Part model, mm, in its own coordinate system. A direction names the side the tool comes from. Coordinates: 2 decimals unless noted, no trailing zeros. Write each loop counter-clockwise with the first axis right and the second up, starting at its lowest first coordinate (ties: lowest second). Pieces come first, ordered by that corner, then holes. Notation, with made-up numbers: (85, -0.75) - (89, -0.75) arc R19 cw to (89, 33.25) - close; hole circle Ø7 at (-27, -29.5). An arc over 180 degrees is marked (long way). Use a Markdown table: item, result.
```python
from build123d import *

# Parameters (mm, degrees)
F1_DEPTH      = 25
F1_DEPTH_BACK = 25
F2_SIZE2      = 5
F2_SIZE       = 1
F3_SIZE2      = 1
F3_SIZE       = 5
F3_2_SIZE2    = 1
F3_2_SIZE     = 5
F3_3_SIZE2    = 1
F3_3_SIZE     = 5
F3_4_SIZE2    = 1
F3_4_SIZE     = 5


with BuildPart() as f1:
    # F0 (on Front) → F1 (new body, two sides)
    with BuildSketch(Plane.XZ) as f1_sk:
        with BuildLine():
            Line((-1.5, -2), (-1.5, -6.0415747119))
            ThreePointArc((-1.5, -6.0415747119), (0, -6.225), (1.5, -6.0415747119))
            Line((1.5, -6.0415747119), (1.5, -2))
            ThreePointArc((1.5, -2), (1.767766953, -1.767766953), (2, -1.5))
            Line((2, -1.5), (6.0415747119, -1.5))
            ThreePointArc((6.0415747119, -1.5), (6.225, 0), (6.0415747119, 1.5))
            Line((6.0415747119, 1.5), (2, 1.5))
            ThreePointArc((2, 1.5), (1.767766953, 1.767766953), (1.5, 2))
            Line((1.5, 2), (1.5, 6.0415747119))
            ThreePointArc((1.5, 6.0415747119), (0, 6.225), (-1.5, 6.0415747119))
            Line((-1.5, 6.0415747119), (-1.5, 2))
            ThreePointArc((-1.5, 2), (-1.767766953, 1.767766953), (-2, 1.5))
            Line((-2, 1.5), (-6.0415747119, 1.5))
            ThreePointArc((-6.0415747119, 1.5), (-6.225, 0), (-6.0415747119, -1.5))
            Line((-6.0415747119, -1.5), (-2, -1.5))
            ThreePointArc((-2, -1.5), (-1.767766953, -1.767766953), (-1.5, -2))
        make_face()
    extrude(amount=F1_DEPTH)
    extrude(f1_sk.sketch, amount=-F1_DEPTH_BACK)

    # F2
    f2_edges = [f1.edges().sort_by_distance(p)[0] for p in [
        (0, -25, 6.225),
        (6.225, -25, 0),
        (0, -25, -6.225),
        (-6.225, -25, 0),
    ]]
    f2_side = f1.faces().sort_by_distance((0, -25, 0))[0]
    chamfer(f2_edges, length=F2_SIZE, length2=F2_SIZE2, reference=f2_side)

    # F3
    f3_edges = [f1.edges().sort_by_distance(p)[0] for p in [
        (0, 25, 6.225),
    ]]
    f3_side = f1.faces().sort_by_distance((0, 2.5, 6.225))[0]
    chamfer(f3_edges, length=F3_SIZE, length2=F3_SIZE2, reference=f3_side)

    # F3#2
    f3_2_edges = [f1.edges().sort_by_distance(p)[0] for p in [
        (6.225, 25, 0),
    ]]
    f3_2_side = f1.faces().sort_by_distance((6.225, 2.5, 0))[0]
    chamfer(f3_2_edges, length=F3_2_SIZE, length2=F3_2_SIZE2, reference=f3_2_side)

    # F3#3
    f3_3_edges = [f1.edges().sort_by_distance(p)[0] for p in [
        (-6.225, 25, 0),
    ]]
    f3_3_side = f1.faces().sort_by_distance((-6.225, 2.5, 0))[0]
    chamfer(f3_3_edges, length=F3_3_SIZE, length2=F3_3_SIZE2, reference=f3_3_side)

    # F3#4
    f3_4_edges = [f1.edges().sort_by_distance(p)[0] for p in [
        (0, 25, -6.225),
    ]]
    f3_4_side = f1.faces().sort_by_distance((0, 2.5, -6.225))[0]
    chamfer(f3_4_edges, length=F3_4_SIZE, length2=F3_4_SIZE2, reference=f3_4_side)


solid = f1.part
```
Item 1: Band-saw the part on B-B, the plane z = -3. Give the cut face in (x, y), then the cut area to 3 significant figures.
From the geometry:
| item | result |
|---|---|
| outline | (-1.5, -25) - (1.5, -25) - (1.5, 25) - (-1.5, 25) - close |
| area | 150 mm^2 |
Item 2: Drop flat-ended pins along their axis: P1, Ø3, axis at y = -4.5, z = 5, coming from the +X side; P2, Ø3, axis at x = 4.5, y = -7, coming from the +Z side; P3, Ø4.5, axis at x = -5, y = 1.5, coming from the -Z side. Give the stop position or say it passes through.
From the geometry:
| item | result |
|---|---|
| P1 | x = 1.5 |
| P2 | z = 1.5 |
| P3 | z = -1.5 |
Item 3: Drill centre lines: probe 1 along Z at (x, y) = (-5.5, 15); probe 2 along X at (y, z) = (12.5, -0.75). Where is each one in solid material? Low to high.
From the geometry:
| item | result |
|---|---|
| probe 1 | -1.5 to 1.5 |
| probe 2 | -6.18 to 6.18 |
Item 4: Band-saw the part on C-C, the plane x = -4.25. Give the cut face in (y, z).
From the geometry:
| item | result |
|---|---|
| outline | (-25, -1.5) - (25, -1.5) - (25, 1.5) - (-25, 1.5) - close |
Item 5: Band-saw the part on D-D, the plane y = 21. Give the cut face in (x, z) (3 decimals).
From the geometry:
| item | result |
|---|---|
| outline | (-5.835, -1.5) - (-2, -1.5) arc R2.5 ccw to (-1.5, -2) - (-1.5, -5.835) arc R6.025 ccw to (1.5, -5.835) - (1.5, -2) arc R2.5 ccw to (2, -1.5) - (5.835, -1.5) arc R6.025 ccw to (5.835, 1.5) - (2, 1.5) arc R2.5 ccw to (1.5, 2) - (1.5, 5.835) arc R6.025 ccw to (-1.5, 5.835) - (-1.5, 2) arc R2.5 ccw to (-2, 1.5) - (-5.835, 1.5) arc R6.025 ccw to start |
Item 6: Band-saw the part on A-A, the plane y = 10.5. Give the cut face in (x, z) (3 decimals), then the cut area to 3 significant figures.
From the geometry:
| item | result |
|---|---|
| outline | (-6.042, -1.5) - (-2, -1.5) arc R2.5 ccw to (-1.5, -2) - (-1.5, -6.042) arc R6.225 ccw to (1.5, -6.042) - (1.5, -2) arc R2.5 ccw to (2, -1.5) - (6.042, -1.5) arc R6.225 ccw to (6.042, 1.5) - (2, 1.5) arc R2.5 ccw to (1.5, 2) - (1.5, 6.042) arc R6.225 ccw to (-1.5, 6.042) - (-1.5, 2) arc R2.5 ccw to (-2, 1.5) - (-6.042, 1.5) arc R6.225 ccw to start |
| area | 65.5 mm^2 |
Item 7: Which spindle directions (+Z, -Z, +X, -X, +Y, -Y) get a long thin tool onto all of the face, cutting with end or side? Do faces 1 (the face through (-1.5, 0, 4)), 2 (the face through (4, 0, 1.5)), 3 (the face through (-1.5, 0, -4)). Say none if no direction does.
From the geometry:
| item | result |
|---|---|
| face 1 | +Z, -X, +Y, -Y |
| face 2 | +Z, +X, +Y, -Y |
| face 3 | -Z, -X, +Y, -Y |
